Verification items for the finished model (mm, model axes). Face numbers are marked on the shaded views. A direction names the side the tool comes from. Coordinates: 2 decimals unless noted, no trailing zeros. Write each loop counter-clockwise with the first axis right and the second up, starting at its lowest first coordinate (ties: lowest second). Pieces come first, ordered by that corner, then holes. Notation, with made-up numbers: M 7,25.25 L 23,25.25 A10 cw 23,42.25 Z; hole C 30,-23 d1. An arc over 180 degrees is marked long. One line per item, written item: value.
Solid Edge part; units mm, degrees
sketch "Sketch1" plane through (0, 0, 0) normal (0, 0, 1) x (1, 0, 0)
  line L0 (2, 0) -> (2, 8)
  line L1 (0, 8) -> (2, 8)
  line L2 (0, 0) -> (0, 8)
  line L3 (0, 0) -> (0, -2.2)
  line L4 (0, -2.2) -> (3.8, -2.2)
  line L5 (3.8, -2.2) -> (3.8, 0)
  line L6 (3.8, 0) -> (2, 0)
revolve "RevolvedProtrusion1" add sketch "Sketch1" angle 360 about axis through (0, 0, 0) along (0, 1, 0)
sketch "Sketch2" plane through (0, 0, 0) normal (1, 0, 0) x (0, 1, 0)
  line L0 (-2.2, 1.9365) -> (-0.9, 1.9365)
  line L1 (0.218, 0) -> (-0.9, 1.9365)
  line L2 (-2.2, 0) -> (0.218, 0)
  line L3 (-2.2, 0) -> (-2.2, 1.9365)
revolve "RevolvedCutout1" cut sketch "Sketch2" angle 360 about axis through (0, -4.5, 0) along (0, 1, 0)
sketch "Sketch3" plane through (0, -2.2, 0) normal (0, -1, 0) x (0, 0, 1)
  circle A0 centre (0, 0) radius 1.9365
  line L0 (-1.25, -0.7217) -> (0, -1.4434)
  line L1 (0, -1.4434) -> (1.25, -0.7217)
  line L2 (1.25, -0.7217) -> (1.25, 0.7217)
  line L3 (1.25, 0.7217) -> (0, 1.4434)
  line L4 (0, 1.4434) -> (-1.25, 0.7217)
  line L5 (-1.25, 0.7217) -> (-1.25, -0.7217)
extrude "Protrusion1" add sketch "Sketch3" against normal up to next
sketch "Sketch4" plane through (0, 0, 0) normal (0, 0, 1) x (1, 0, 0)
  line L0 (-1.4434, -2.2) -> (0, -2.2)
  line L1 (0, -2.2) -> (0, -1.8132)
  line L2 (0, -1.8132) -> (-1.4434, -2.2)
revolve "RevolvedCutout2" cut sketch "Sketch4" angle 360 about axis through (0, -4.5, 0) along (0, 1, 0)
fillet "Round1" radius 0.2 1 edges at (0, 0, -2)
chamfer "倒斜角_2" distance 0.2667 angle 45 1 edges at (0, 8, -2)
cosmetic_thread "螺纹_3" thread depth 6.6
sketch "Sketch5" plane through (0, 0, 0) normal (0, 0, 1) x (1, 0, 0)
  arc A0 (-1.9153, -2.2) -> (-3.8, 0) centre (-1.5736, 0) cw
revolve "RevolvedCutout3" cut sketch "Sketch5" angle 360 about axis through (0, 0, 0) along (0, -1, 0) material side at (-3.3024, -1.481, 0)
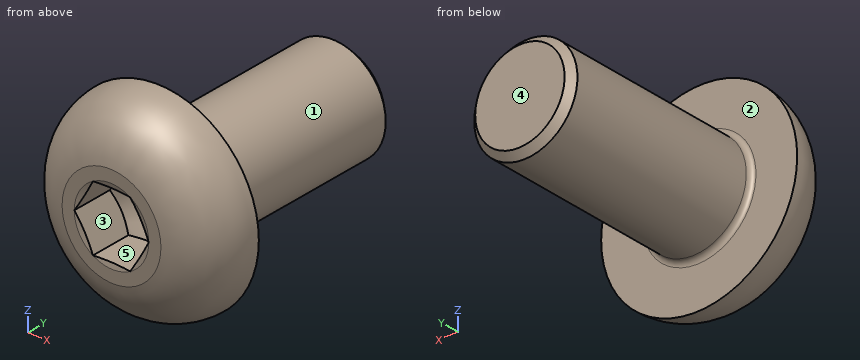
Item 1: Scan lines: line 1 (X direction, y = -0.75, z = -1); line 2 (Z direction, x = -1, y = 6.25); line 3 (Z direction, x = 1.75, y = -1.5). Record each from-to range of solid material in increasing order.
The answers:
line 1: x = -3.53 to -0.87, 0.87 to 3.53
line 2: z = -1.73 to 1.73
line 3: z = -2.7 to 2.7
Item 2: Go/stop test with flat-tipped pins: P1, Ø4, axis at y = 7, z = 2, coming from the -X side; P2, Ø4, axis at x = 2, y = 1, coming from the +Z side; P3, Ø3, axis at y = 5, z = 2.5, coming from the +X side. Record where each tip stops, or that it passes through.
The answers:
P1: stops at x = -2
P2: stops at z = 3.79
P3: stops at x = 1.73
Item 3: Cross-section at A-A, the plane y = 1.5. Enter the section's corners in (x, z), and give its area (3 significant figures).
The answers:
outline: C 0,0 d4
area: 12.6 mm²
Item 4: Draft check along Z on the marked faces 1, 2 and 3. Enter one of: released by +Z, released by -Z, zero draft, split by the parting line, or undercut.
The answers:
face 1: split by the parting line
face 2: zero draft
face 3: undercut
Item 5: Access from +Z, -Z, +X, -X, +Y, -Y to the whole of each face (thin tool, end or side, straight path). Record for the marked faces 4 and 5.
The answers:
face 4: +Z, -Z, +X, -X, +Y
face 5: -Y
